from build123d import *

# Parameters (mm, degrees)
SKETCH1_W                               = 50
SKETCH1_H                               = 30
BOSS_EXTRUDE1_DEPTH                     = 10
BOSS_EXTRUDE3_DEPTH                     = 10
CBORE_FOR_M5_HEX_HEAD_BOLT1_D           = 5.3
CBORE_FOR_M5_HEX_HEAD_BOLT1_CBORE_D     = 12.24
CBORE_FOR_M5_HEX_HEAD_BOLT1_CBORE_DEPTH = 0.5
FILLET1_SIZE                            = 10
SKETCH15_R                              = 9.55
CUT_EXTRUDE1_DEPTH                      = 6
SKETCH16_R                              = 7.55
CUT_EXTRUDE2_DEPTH                      = 52.429563531


with BuildPart() as part:
    # Sketch1 → Boss-Extrude1 (new body)
    with BuildSketch(Plane.XY):
        Rectangle(SKETCH1_W, SKETCH1_H)
    extrude(amount=BOSS_EXTRUDE1_DEPTH)

    # Sketch8 → Boss-Extrude3 (add)
    with BuildSketch(Plane(origin=(0, 15, 0), x_dir=(1, 0, 0), z_dir=(0, 1, 0))):
        with BuildLine():
            Line((-25, -10), (-12.942664449, -30.582047017))
            ThreePointArc((-12.942664449, -30.582047017), (0, -38), (12.942664449, -30.582047017))
            Line((12.942664449, -30.582047017), (25, -10))
            Line((25, -10), (-25, -10))
        make_face()
    extrude(amount=-BOSS_EXTRUDE3_DEPTH)

    # CBORE for M5 Hex Head Bolt1 (through all)
    with Locations(Plane.XY.offset(10)):
        with Locations((12.5, -3), (-12.5, -3)):
            CounterBoreHole(CBORE_FOR_M5_HEX_HEAD_BOLT1_D / 2, CBORE_FOR_M5_HEX_HEAD_BOLT1_CBORE_D / 2, CBORE_FOR_M5_HEX_HEAD_BOLT1_CBORE_DEPTH)

    # Fillet1
    # a fillet whose section is not a circle: 10 mm, written as the material it adds along each edge
    with BuildSketch(Plane(origin=(50, 5, 10), x_dir=(0, -1, 0), z_dir=(-1, 0, 0))) as fillet1_piece_1_section:
        with BuildLine():
            add(Edge.make_bspline([(FILLET1_SIZE, 0), (FILLET1_SIZE * 0.831801948466, 0), (FILLET1_SIZE * 0.663603896932, 0), (FILLET1_SIZE * 0.292893218813, FILLET1_SIZE * 0.0716919198361), (FILLET1_SIZE * 0.0716919198361, FILLET1_SIZE * 0.292893218813), (0, FILLET1_SIZE * 0.663603896932), (0, FILLET1_SIZE * 0.831801948466), (0, FILLET1_SIZE)], knots=[0, 0, 0, 0, 0, 0, 0.5, 0.5, 1, 1, 1, 1, 1, 1], degree=5))
            Line((0, FILLET1_SIZE), (0, 0))
            Line((0, 0), (FILLET1_SIZE, 0))
        make_face()
    fillet1_piece_1 = extrude(amount=100, mode=Mode.PRIVATE)
    fillet1_piece_1 = split(fillet1_piece_1, bisect_by=Plane(origin=(-5.837521011, 5, 42.710630125), z_dir=(0.8628442965853785, 0, -0.5054698011257285)), keep=Keep.TOP, mode=Mode.PRIVATE)
    fillet1_piece_1 = split(fillet1_piece_1, bisect_by=Plane(origin=(31.387492996, 5, -0.903543375), z_dir=(-0.8628442965853789, 0, -0.5054698011257279)), keep=Keep.TOP, mode=Mode.PRIVATE)
    fillet1_piece_1 = fillet1_piece_1 - Plane(origin=(12.5, -3, 10), x_dir=(1, 0, 0), z_dir=(0, 0, 1)) * Cylinder(6.12, 240, mode=Mode.PRIVATE)
    fillet1_piece_1 = fillet1_piece_1 - Plane(origin=(-12.5, -3, 10), x_dir=(1, 0, 0), z_dir=(0, 0, 1)) * Cylinder(6.12, 240, mode=Mode.PRIVATE)
    add(fillet1_piece_1)

    # Sketch15 → Cut-Extrude1 (cut)
    with BuildSketch(Plane(origin=(0, 15, 0), x_dir=(1, 0, 0), z_dir=(0, 1, 0))):
        with Locations(Location((0, -23, 0), (0, 0, 270))):
            Circle(SKETCH15_R)
    extrude(amount=-CUT_EXTRUDE1_DEPTH, mode=Mode.SUBTRACT)

    # Sketch16 → Cut-Extrude2 (cut, through all)
    with BuildSketch(Plane(origin=(0, 9, 0), x_dir=(1, 0, 0), z_dir=(0, 1, 0))):
        with Locations(Location((0, -23, 0), (0, 0, 270))):
            Circle(SKETCH16_R)
    extrude(amount=-CUT_EXTRUDE2_DEPTH, mode=Mode.SUBTRACT)


solid = part.part
Design review of the part built by this model. Coordinates are the model's own, in mm. A direction names the side the tool comes from. Round coordinates to 2 decimals unless told otherwise and drop trailing zeros. Write each loop counter-clockwise with the first axis right and the second up, starting at its lowest first coordinate (ties: lowest second). Pieces come first, ordered by that corner, then holes. Notation, with made-up numbers: (-16.75, 8) -> (37.25, 8) arc R7 ccw to (37.25, 20) -> close; hole circle Ø9 at (46, -18.5). An arc over 180 degrees is marked (long way). One line per item, written item: value. Start each with the question number.
Q1. Insertion check: P1, Ø15.5, axis at x = 3, z = 24.5, coming from the +Y side; P2, Ø3.5, axis at x = -13, y = -1, coming from the +Z side; P3, Ø1, axis at x = 12.5, z = 28.5, coming from the -Y side; P4, Ø4, axis at x = 0.5, y = -1, coming from the +Z side. Each pin has a flat end and moves straight along its axis. Give the tip position at first contact, or say it passes through.
Q2. Add section C-C (z = 28). Give the boundary of the cut face in (x, y).
Q3. To check wall thickness, follow probe 1 along X at (y, z) = (-3, 9.75); probe 2 along X at (y, z) = (11, 23.5); probe 3 along Y at (x, z) = (13, 30). State the ranges of each line that lie inside material, in increasing order.
Q4. Tool access review of faces 4 (the face through (8, 9, 24)), 5 (the face through (-9.9, -4.3, 9.5)), 6 (the face through (0, 5, 31)): name each direction out of +Z, -Z, +X, -X, +Y, -Y from which nothing blocks a thin tool from reaching the whole face with its end or side.
Q5. Add section B-B (z = 6.5). Give the boundary of the cut face in (x, y), then the cut area to 3 significant figures.
Q6. Add section A-A (y = 10.75). Give the boundary of the cut face in (x, z).
Q7. Add section D-D (y = -3). State how many separate pieces and enclosed holes the cut face has, then the cut area to 3 significant figures.
Q8. The part is to be moulded in two halves that separate along X. For faces 1 (the face through (-25, 0, 5)), 2 (the face through (0, 0, 0)), 3 (the face through (-3.66, 12.04, 31.82)), say which applies: pulls with the +X half, pulls with the -X half, needs draft (parallel to the pull), parting line crosses it, or undercut.
Response:
1. P1: stops at y = 15
1. P2: stops at z = 9.5
1. P3: stops at y = 5
1. P4: stops at z = 10.95
2. outline: (-14.46, 5) -> (-5.66, 5) -> (-5.66, 9) -> (-8.14, 9) -> (-8.14, 15) -> (-14.46, 15) -> close; (5.66, 5) -> (14.46, 5) -> (14.46, 15) -> (8.14, 15) -> (8.14, 9) -> (5.66, 9) -> close
3. probe 1: x = -25 to -18.62, -6.38 to 6.38, 18.62 to 25
3. probe 2: x = -17.09 to -9.54, 9.54 to 17.09
3. probe 3: y = 5 to 15
4. face 4: +Y
4. face 5: +Z
4. face 6: +Z, +X, -X, -Y
5. outline: (-25, -15) -> (25, -15) -> (25, 15) -> (-25, 15) -> close; hole circle Ø5.3 at (-12.5, -3); hole circle Ø5.3 at (12.5, -3)
5. area: 1,460 mm^2
6. outline: (-25, 0) -> (25, 0) -> (25, 10) -> (12.94, 30.58) arc R15 ccw to (-12.94, 30.58) -> (-25, 10) -> close; hole circle Ø19.1 at (0, 23)
7. separate pieces: 3
7. enclosed holes: 0
7. area: 388 mm^2
8. face 1: pulls with the -X half
8. face 2: needs draft
8. face 3: undercut
